Could you check a few things on this model? Use its own coordinates, in mm. A direction names the side the tool comes from. Coordinates: 2 decimals unless noted, no trailing zeros. Order: outer loops, then holes, each group sorted by start corner. A loop starts at its lowest first (then second) coordinate and runs counter-clockwise, first axis right, second up. Notation, with made-up numbers: (74.5, 39) -> (95.5, 39) arc R35 ccw to (95.5, 76) -> close; hole circle Ø5 at (-10, 41). An arc over 180 degrees is marked (long way). Return JSON: item names as keys, results as strings. Group by question number.
from build123d import *

# Parameters (mm, degrees)
SKETCH_1_W      = 98
SKETCH_1_H      = 60
SKETCH_1_R      = 1.6
EXTRUDE_1_DEPTH = 3
FILLET_4_R      = 2


with BuildPart() as part:
    # 草图1 → 凸台-拉伸1 (new body)
    with BuildSketch(Plane.XY):
        with Locations((49, 30)):
            Rectangle(SKETCH_1_W, SKETCH_1_H)
        with Locations((8, 8)):
            Circle(SKETCH_1_R, mode=Mode.SUBTRACT)
        with Locations(Location((90, 8, 0), (0, 0, 180))):
            Circle(SKETCH_1_R, mode=Mode.SUBTRACT)
        with Locations((90, 52)):
            Circle(SKETCH_1_R, mode=Mode.SUBTRACT)
        with Locations(Location((8, 52, 0), (0, 0, 180))):
            Circle(SKETCH_1_R, mode=Mode.SUBTRACT)
        Polygon((49, 56.461504081), (39.652852225, 32.437112926), (49, 13.645736298), (58.347147775, 32.437112926), align=None, mode=Mode.SUBTRACT)
        Polygon((32.684961024, 14.527976606), (46.19127915, 14.527976606), (38.625617, 29.796874275), align=None, mode=Mode.SUBTRACT)
        Polygon((65.315038976, 14.527976606), (59.374383, 29.796874275), (51.80872085, 14.527976606), align=None, mode=Mode.SUBTRACT)
        Polygon((51.754435798, 55.675997791), (61.074674823, 31.720768521), (81.417430018, 55.675997791), align=None, mode=Mode.SUBTRACT)
        Polygon((83.46136082, 55.573734568), (61.744172649, 30), (90.184817286, 30), align=None, mode=Mode.SUBTRACT)
        Polygon((62.560585094, 27.901625993), (68.503620332, 12.626613057), (83.282124763, 5.998312223), (93.091894324, 18.94247075), (90.736489794, 27.901625993), align=None, mode=Mode.SUBTRACT)
        Polygon((34.516229814, 12.626613057), (63.483770186, 12.626613057), (84.583930387, 3.16298904), (13.416069613, 3.16298904), align=None, mode=Mode.SUBTRACT)
        Polygon((14.717875237, 5.998312223), (4.908105676, 18.94247075), (7.263510206, 27.901625993), (35.439414906, 27.901625993), (29.496379668, 12.626613057), align=None, mode=Mode.SUBTRACT)
        Polygon((14.53863918, 55.573734568), (36.255827351, 30), (7.815182714, 30), align=None, mode=Mode.SUBTRACT)
        Polygon((36.925325177, 31.720768521), (16.582569982, 55.675997791), (46.245564202, 55.675997791), align=None, mode=Mode.SUBTRACT)
        Polygon((2.839889493, 48.591962143), (11.02417284, 48.591962143), (2.839889493, 19.702141439), align=None, mode=Mode.SUBTRACT)
        Polygon((86.97582716, 48.591962143), (95.160110507, 19.702141439), (95.160110507, 48.591962143), align=None, mode=Mode.SUBTRACT)
    extrude(amount=EXTRUDE_1_DEPTH)

    # 圆角4
    fillet_4_edges = [part.edges().sort_by_distance(p)[0] for p in [
        (90.736489794, 27.901625993, 1.5),
        (62.560585094, 27.901625993, 1.5),
        (2.839889493, 48.591962143, 1.5),
        (2.839889493, 19.702141439, 1.5),
        (11.02417284, 48.591962143, 1.5),
        (95.160110507, 48.591962143, 1.5),
        (86.97582716, 48.591962143, 1.5),
        (95.160110507, 19.702141439, 1.5),
        (35.439414906, 27.901625993, 1.5),
        (7.263510206, 27.901625993, 1.5),
        (4.908105676, 18.94247075, 1.5),
        (14.717875237, 5.998312223, 1.5),
        (29.496379668, 12.626613057, 1.5),
        (14.53863918, 55.573734568, 1.5),
        (7.815182714, 30, 1.5),
        (36.255827351, 30, 1.5),
        (36.925325177, 31.720768521, 1.5),
        (46.245564202, 55.675997791, 1.5),
        (16.582569982, 55.675997791, 1.5),
        (58.347147775, 32.437112926, 1.5),
        (49, 56.461504081, 1.5),
        (39.652852225, 32.437112926, 1.5),
        (49, 13.645736298, 1.5),
        (38.625617, 29.796874275, 1.5),
        (32.684961024, 14.527976606, 1.5),
        (46.19127915, 14.527976606, 1.5),
        (81.417430018, 55.675997791, 1.5),
        (51.754435798, 55.675997791, 1.5),
        (61.074674823, 31.720768521, 1.5),
        (51.80872085, 14.527976606, 1.5),
        (65.315038976, 14.527976606, 1.5),
        (59.374383, 29.796874275, 1.5),
        (90.184817286, 30, 1.5),
        (83.46136082, 55.573734568, 1.5),
        (61.744172649, 30, 1.5),
        (34.516229814, 12.626613057, 1.5),
        (13.416069613, 3.16298904, 1.5),
        (84.583930387, 3.16298904, 1.5),
        (63.483770186, 12.626613057, 1.5),
        (68.503620332, 12.626613057, 1.5),
        (83.282124763, 5.998312223, 1.5),
        (93.091894324, 18.94247075, 1.5),
    ]]
    fillet(fillet_4_edges, radius=FILLET_4_R)


solid = part.part
Q1. On a 3-axis mill with a long thin cutter (end or side, diameter ignored), from which of +Z, -Z, +X, -X, +Y, -Y can I reach the whole of each face in a straight line? I mean faces 3 (the flat face through (42, 26, 3)), 4 (the cylindrical face through (78.9, 54.54, 1.52)). Say none if no direction works.
Q2. I need wall thicknesses on line 1 along Y through (x, z) = (74, 2.95); line 2 along X through (y, z) = (55.5, 2.2); line 3 along X through (y, z) = (49.5, 2.3). Which ranges of each line are inside material? Lowest first, please. Write a range as from..to.
Q3. We'd pull the mould along Y, two halves only. Please class faces 1 (the flat face through (0, 30, 1)), 2 (the flat face through (75.45, 9.51, 1.48)): pulls with the +Y half, pulls with the -Y half, needs draft (parallel to the pull), parting line crosses it, or undercut.
Q4. I'm going to push flat-ended pins straight in: pin 1 Ø1.5 at (x, z) = (90.5, 1.5) entering from -Y; pin 2 Ø3 at (x, y) = (8, 8) entering from -Z. Where does each tip first touch, or does it pass through?
Q5. I want a section at A-A on y = 5. Please give me the cut outline in (x, z), and give its area (3 significant figures).
Q6. I want a section at B-B on z = 1.6. State how many separate pieces and enclosed holes the cut face has, and give its area (3 significant figures).
Response values:
{
 "1": {"face 3": "+Z, +X, -X, +Y, -Y", "face 4": "+Z, -Z"},
 "2": {"line 1": "y = 0..3.16, 7.91..10.16, 27.9..30, 44.43..46.94, 55.68..60", "line 2": "x = 0..20.08, 44.14..53.86, 77.92..98", "line 3": "x = 0..12.94, 19.7..21.83, 43.84..46.29, 51.71..54.16, 76.17..78.3, 85.06..98"},
 "3": {"face 1": "needs draft", "face 2": "undercut"},
 "4": {"pin 1": "stops at y = 0", "pin 2": "passes through"},
 "5": {"outline": "(0, 0) -> (20.77, 0) -> (20.77, 3) -> (0, 3) -> close; (77.23, 0) -> (98, 0) -> (98, 3) -> (77.23, 3) -> close", "area": "125 mm²"},
 "6": {"separate pieces": "1", "enclosed holes": "16", "area": "2,320 mm²"}
}
